Can you work these out from the model? Positions are in its coordinate system, mm. A direction names the side the tool comes from. Coordinates: 2 decimals unless noted, no trailing zeros. Loops run counter-clockwise (first coordinate to the right, second up) from the corner with the lowest first, then second, coordinate; pieces in that order, holes last.
```python
from build123d import *

# Parameters (mm, degrees)
SKETCH_1_W                 = 75
SKETCH_1_H                 = 47
SKETCH_1_R                 = 10.25
SKETCH_1_R_2               = 4.39
EXTRUDE_746_DEPTH          = 3
HOLE_WIZARD_M3_AT_2_COUNT  = 2
HOLE_WIZARD_M3_AT_2_PITCH  = 30
HOLE_WIZARD_M3_AT_3_COUNT  = 2
HOLE_WIZARD_M3_AT_3_PITCH  = 30
HOLE_WIZARD_M3_AT_4_COUNT  = 2
HOLE_WIZARD_M3_AT_4_PITCH  = 40.75
HOLE_WIZARD_M3_AT_5_COUNT  = 2
HOLE_WIZARD_M3_AT_5_PITCH  = 50.602000949
HOLE_WIZARD_M3_AT_6_COUNT  = 2
HOLE_WIZARD_M3_AT_6_PITCH  = 50.602000949
HOLE_WIZARD_M3_AT_7_COUNT  = 2
HOLE_WIZARD_M3_AT_7_PITCH  = 35.472700771
HOLE_WIZARD_M3_AT_8_COUNT  = 2
HOLE_WIZARD_M3_AT_8_PITCH  = 35.472700771
HOLE_WIZARD_M3_AT_9_COUNT  = 2
HOLE_WIZARD_M3_AT_9_PITCH  = 46.549033287
HOLE_WIZARD_M3_AT_10_COUNT = 2
HOLE_WIZARD_M3_AT_10_PITCH = 46.549033287
CHAMFER_1_SIZE             = 0.5
SKETCH_6_W                 = 17
SKETCH_6_H                 = 5.5
CUT_EXTRUDE_1_DEPTH        = 61.201744161
FILLET_1_R                 = 2
HOLE_WIZARD_M21_D          = 1.6
SKETCH_10_R                = 7.5
SKETCH_10_R_2              = 4.39
EXTRUDE_1_DEPTH            = 7
CHAMFER_2_SIZE             = 1


with BuildPart() as part:
    # Эскиз1 → Extrude 746 (new body)
    with BuildSketch(Plane(origin=(0, 0, 0), x_dir=(1, 0, 0), z_dir=(0, 1, 0))):
        with Locations((0, -23.5)):
            Rectangle(SKETCH_1_W, SKETCH_1_H)
        with Locations(Location((18, -29, 0), (0, 0, 270))):
            Circle(SKETCH_1_R, mode=Mode.SUBTRACT)
        with Locations(Location((-18, -29, 0), (0, 0, 270))):
            Circle(SKETCH_1_R, mode=Mode.SUBTRACT)
        with Locations(Location((0, -29, 0), (0, 0, 270))):
            Circle(SKETCH_1_R_2, mode=Mode.SUBTRACT)
    extrude(amount=EXTRUDE_746_DEPTH)

    # Эскиз3 → Крепление стенок M3 (revolve, cut)
    with BuildSketch(Plane(origin=(0, 0, 44.5), x_dir=(0, 0, -1), z_dir=(1, 0, 0))):
        Polygon((0, 0), (0, 3), (1.7, 3), (1.7, 1.45), (3.15, 0), align=None)
    hole_wizard_m3 = revolve(axis=Axis((0, -6.35, 44.5), (0, 1, 0)), mode=Mode.SUBTRACT)

    # Крепление стенок M3 at 2: Крепление стенок M3 ×2
    with Locations(*[(i * HOLE_WIZARD_M3_AT_2_PITCH, 0, 0) for i in range(1, HOLE_WIZARD_M3_AT_2_COUNT)]):
        add(hole_wizard_m3, mode=Mode.SUBTRACT)

    # Крепление стенок M3 at 3: Крепление стенок M3 ×2
    with Locations(*[(-i * HOLE_WIZARD_M3_AT_3_PITCH, 0, 0) for i in range(1, HOLE_WIZARD_M3_AT_3_COUNT)]):
        add(hole_wizard_m3, mode=Mode.SUBTRACT)

    # Крепление стенок M3 at 4: Крепление стенок M3 ×2
    with Locations(*[(0, 0, -i * HOLE_WIZARD_M3_AT_4_PITCH) for i in range(1, HOLE_WIZARD_M3_AT_4_COUNT)]):
        add(hole_wizard_m3, mode=Mode.SUBTRACT)

    # Крепление стенок M3 at 5: Крепление стенок M3 ×2
    with Locations(*[Vector(-0.5928619311020034, 0, -0.8053041230802209) * (i * HOLE_WIZARD_M3_AT_5_PITCH) for i in range(1, HOLE_WIZARD_M3_AT_5_COUNT)]):
        add(hole_wizard_m3, mode=Mode.SUBTRACT)

    # Крепление стенок M3 at 6: Крепление стенок M3 ×2
    with Locations(*[Vector(0.5928619311020034, 0, -0.8053041230802209) * (i * HOLE_WIZARD_M3_AT_6_PITCH) for i in range(1, HOLE_WIZARD_M3_AT_6_COUNT)]):
        add(hole_wizard_m3, mode=Mode.SUBTRACT)

    # Крепление стенок M3 at 7: Крепление стенок M3 ×2
    with Locations(*[Vector(-0.972578891654415, 0, -0.23257321322170757) * (i * HOLE_WIZARD_M3_AT_7_PITCH) for i in range(1, HOLE_WIZARD_M3_AT_7_COUNT)]):
        add(hole_wizard_m3, mode=Mode.SUBTRACT)

    # Крепление стенок M3 at 8: Крепление стенок M3 ×2
    with Locations(*[Vector(0.972578891654415, 0, -0.23257321322170757) * (i * HOLE_WIZARD_M3_AT_8_PITCH) for i in range(1, HOLE_WIZARD_M3_AT_8_COUNT)]):
        add(hole_wizard_m3, mode=Mode.SUBTRACT)

    # Крепление стенок M3 at 9: Крепление стенок M3 ×2
    with Locations(*[Vector(0.7411539523694183, 0, -0.6713351017838932) * (i * HOLE_WIZARD_M3_AT_9_PITCH) for i in range(1, HOLE_WIZARD_M3_AT_9_COUNT)]):
        add(hole_wizard_m3, mode=Mode.SUBTRACT)

    # Крепление стенок M3 at 10: Крепление стенок M3 ×2
    with Locations(*[Vector(-0.7411539523694182, 0, -0.6713351017838932) * (i * HOLE_WIZARD_M3_AT_10_PITCH) for i in range(1, HOLE_WIZARD_M3_AT_10_COUNT)]):
        add(hole_wizard_m3, mode=Mode.SUBTRACT)

    # Фаска1
    chamfer_1_edges = [part.edges().sort_by_distance(p)[0] for p in [
        (0, 0, 24.61),
        (18, 0, 18.75),
        (-18, 0, 18.75),
    ]]
    chamfer(chamfer_1_edges, length=CHAMFER_1_SIZE)

    # Эскиз6 → Вырез-Вытянуть1 (cut, through all)
    with BuildSketch(Plane.XZ):
        with Locations((0, 12.25)):
            Rectangle(SKETCH_6_W, SKETCH_6_H)
    extrude(amount=-CUT_EXTRUDE_1_DEPTH, mode=Mode.SUBTRACT)

    # Скругление1
    fillet_1_edges = [part.edges().sort_by_distance(p)[0] for p in [
        (-8.5, 1.5, 9.5),
        (-8.5, 1.5, 15),
        (8.5, 1.5, 15),
        (8.5, 1.5, 9.5),
    ]]
    fillet(fillet_1_edges, radius=FILLET_1_R)

    # Отверстие обработанное метчиком M21 (through all)
    with Locations(Plane(origin=(0, 0, 0), x_dir=(-1, 0, 0), z_dir=(0, -1, 0))):
        with Locations((27.8, -14.8), (-27.8, -14.8)):
            Hole(HOLE_WIZARD_M21_D / 2)

    # Эскиз10 → Бобышка-Вытянуть1 (add)
    with BuildSketch(Plane(origin=(0, 3, 0), x_dir=(1, 0, 0), z_dir=(0, 1, 0))):
        with Locations(Location((0, -29, 0), (0, 0, 270))):
            Circle(SKETCH_10_R)
        with Locations(Location((0, -29, 0), (0, 0, 270))):
            Circle(SKETCH_10_R_2, mode=Mode.SUBTRACT)
    extrude(amount=EXTRUDE_1_DEPTH)

    # Фаска2
    chamfer_2_edges = [part.edges().sort_by_distance(p)[0] for p in [
        (0, 10, 21.5),
    ]]
    chamfer(chamfer_2_edges, length=CHAMFER_2_SIZE)


solid = part.part
```
Item 1: Suppose I cut it at C-C, the plane x = -18. Please give me the cut outline in (y, z), plus the area to 4 significant figures.
Results are:
outline: (0, 0) - (3, 0) - (3, 18.75) - (0.5, 18.75) - (0, 18.25) - close; (0, 39.75) - (0.5, 39.25) - (3, 39.25) - (3, 47) - (0, 47) - close
area: 79.25 mm2
Item 2: Suppose I cut it at A-A, the plane x = 30. Please give me the cut outline in (y, z).
Results are:
outline: (0, 0) - (3, 0) - (3, 2.05) - (1.45, 2.05) - (0, 0.6) - close; (0, 6.9) - (1.45, 5.45) - (3, 5.45) - (3, 42.8) - (1.45, 42.8) - (0, 41.35) - close; (0.65, 47) - (1.45, 46.2) - (3, 46.2) - (3, 47) - close
Item 3: I'm going to push flat-ended pins straight in: P1, Ø6, axis at y = 6.5, z = 24.5, coming from the -X side; P2, Ø8, axis at x = -11.5, z = 33, coming from the -Y side; P3, Ø2, axis at x = 27.8, z = 14.8, coming from the +Y side; P4, Ø1.5, axis at y = 8, z = 22.5, coming from the +X side. Where does each tip first touch, or does it pass through?
Results are:
P1: stops at x = -7.35
P2: stops at y = 0
P3: stops at y = 3
P4: stops at x = 4.82
Item 4: We'd pull the mould along X, two halves only. Please class faces 1 (the face through (0, 1, 15)), 2 (the face through (0.33, 5.958, 21.507)), 3 (the face through (-1, 1, 0)): +X half, -X half, draft (parallel to the pull), parting line (faces both ways), or undercut.
Results are:
face 1: undercut
face 2: parting line
face 3: draft
Item 5: Suppose I cut it at D-D, the plane y = 7. Please give me the cut outline in (x, z), plus the area to 3 significant figures.
Results are:
outline: circle Ø15 at (0, 29); hole circle Ø8.78 at (0, 29)
area: 116 mm2
Item 6: I need wall thicknesses on line 1 along X through (y, z) = (2.1, 29); line 2 along Z through (x, y) = (34.5, 2.65); line 3 along Z through (x, y) = (-30, 2.25). Which ranges of each line are inside material? Lowest first, please.
Results are:
line 1: x = -37.5 to -28.25, -7.75 to -4.39, 4.39 to 7.75, 28.25 to 37.5
line 2: z = 0 to 11.55, 14.95 to 34.55, 37.95 to 47
line 3: z = 0 to 2.05, 5.45 to 42.8, 46.2 to 47
Item 7: On a 3-axis mill with a long thin cutter (end or side, diameter ignored), from which of +Z, -Z, +X, -X, +Y, -Y can I reach the whole of each face in a straight line? I mean faces 4 (the face through (-1, 0, 18)), 5 (the face through (0, 1, 9.5)). Say none if no direction works.
Results are:
face 4: +Z, -Z, +X, -X, -Y
face 5: +Y, -Y
Item 8: Suppose I cut it at B-B, the plane z = 3.75. Please give me the cut outline in (x, y).
Results are:
outline: (-37.5, 0) - (-33.15, 0) - (-31.7, 1.45) - (-31.7, 3) - (-37.5, 3) - close; (-28.3, 1.45) - (-26.85, 0) - (-3.15, 0) - (-1.7, 1.45) - (-1.7, 3) - (-28.3, 3) - close; (1.7, 1.45) - (3.15, 0) - (26.85, 0) - (28.3, 1.45) - (28.3, 3) - (1.7, 3) - close; (31.7, 1.45) - (33.15, 0) - (37.5, 0) - (37.5, 3) - (31.7, 3) - close
